from build123d import *

# Parameters (mm, degrees)
SKETCH1_W           = 177.8
SKETCH1_H           = 19.05
BOSS_EXTRUDE1_DEPTH = 3.048
CUT_EXTRUDE1_DEPTH  = 179.843598722
BOSS_EXTRUDE2_DEPTH = 3.048
FILLET1_R           = 1.5875
FILLET2_R           = 0.79375


with BuildPart() as part:
    # Sketch1 → Boss-Extrude1 (new body)
    with BuildSketch(Plane.XY):
        with Locations((-88.9, 9.525)):
            Rectangle(SKETCH1_W, SKETCH1_H)
    extrude(amount=BOSS_EXTRUDE1_DEPTH)

    # Sketch2 → Cut-Extrude1 (cut, through all)
    with BuildSketch(Plane.XY.offset(3.048)):
        with BuildLine():
            Line((-11.1125, 6.35), (-20.6375, 6.35))
            ThreePointArc((-20.6375, 6.35), (-23.8125, 9.525), (-20.6375, 12.7))
            Line((-20.6375, 12.7), (-11.1125, 12.7))
            ThreePointArc((-11.1125, 12.7), (-7.9375, 9.525), (-11.1125, 6.35))
        make_face()
        with BuildLine():
            Line((-36.5125, 6.35), (-46.0375, 6.35))
            ThreePointArc((-46.0375, 6.35), (-49.2125, 9.525), (-46.0375, 12.7))
            Line((-46.0375, 12.7), (-36.5125, 12.7))
            ThreePointArc((-36.5125, 12.7), (-33.3375, 9.525), (-36.5125, 6.35))
        make_face()
        with BuildLine():
            Line((-61.9125, 6.35), (-71.4375, 6.35))
            ThreePointArc((-71.4375, 6.35), (-74.6125, 9.525), (-71.4375, 12.7))
            Line((-71.4375, 12.7), (-61.9125, 12.7))
            ThreePointArc((-61.9125, 12.7), (-58.7375, 9.525), (-61.9125, 6.35))
        make_face()
        with BuildLine():
            Line((-87.3125, 6.35), (-96.8375, 6.35))
            ThreePointArc((-96.8375, 6.35), (-100.0125, 9.525), (-96.8375, 12.7))
            Line((-96.8375, 12.7), (-87.3125, 12.7))
            ThreePointArc((-87.3125, 12.7), (-84.1375, 9.525), (-87.3125, 6.35))
        make_face()
        with BuildLine():
            Line((-112.7125, 6.35), (-122.2375, 6.35))
            ThreePointArc((-122.2375, 6.35), (-125.4125, 9.525), (-122.2375, 12.7))
            Line((-122.2375, 12.7), (-112.7125, 12.7))
            ThreePointArc((-112.7125, 12.7), (-109.5375, 9.525), (-112.7125, 6.35))
        make_face()
        with BuildLine():
            Line((-138.1125, 6.35), (-147.6375, 6.35))
            ThreePointArc((-147.6375, 6.35), (-150.8125, 9.525), (-147.6375, 12.7))
            Line((-147.6375, 12.7), (-138.1125, 12.7))
            ThreePointArc((-138.1125, 12.7), (-134.9375, 9.525), (-138.1125, 6.35))
        make_face()
    extrude(amount=-CUT_EXTRUDE1_DEPTH, mode=Mode.SUBTRACT)

    # Sketch3 → Boss-Extrude2 (add)
    with BuildSketch(Plane(origin=(0, 0, 0), x_dir=(-1, 0, 0), z_dir=(0, 0, -1))):
        Polygon((177.8, 0), (190.5, 0), (190.5, 11.176), (177.8, 19.05), align=None)
    extrude(amount=-BOSS_EXTRUDE2_DEPTH)

    # Fillet1
    fillet1_edges = [part.edges().sort_by_distance(p)[0] for p in [
        (-190.5, 0, 1.524),
        (-190.5, 11.176, 1.524),
        (-177.8, 19.05, 1.524),
    ]]
    fillet(fillet1_edges, radius=FILLET1_R)

    # Fillet2
    fillet2_edges = [part.edges().sort_by_distance(p)[0] for p in [
        (0, 0, 1.524),
        (0, 19.05, 1.524),
    ]]
    fillet(fillet2_edges, radius=FILLET2_R)


solid = part.part
Design review of the part built by this model. Coordinates are the model's own, in mm. A direction names the side the tool comes from. Round coordinates to 2 decimals unless told otherwise and drop trailing zeros. Loops run counter-clockwise (first coordinate to the right, second up) from the corner with the lowest first, then second, coordinate; pieces in that order, holes last. Notation, with made-up numbers: M 11,41.5 L 28,41.5 A25 ccw 28,70.5 Z; hole C 37,79.5 d10. An arc over 180 degrees is marked long. Answer as a JSON object with one key per item and string values.
Item 1: We need section C-C on y = 16.25. Give the boundary of the cut face in (x, z).
Answer sheet:
{"outline": "M -182.32,0 L 0,0 L 0,3.05 L -182.32,3.05 Z"}
Item 2: We need section A-A on x = -143. Give the boundary of the cut face in (y, z), and give its area (3 significant figures).
Answer sheet:
{"outline": "M 0,0 L 6.35,0 L 6.35,3.05 L 0,3.05 Z; M 12.7,0 L 19.05,0 L 19.05,3.05 L 12.7,3.05 Z", "area": "38.7 mm^2"}
Item 3: We need section B-B on z = 0.6. State how many separate pieces and enclosed holes the cut face has, and give its area (3 significant figures).
Answer sheet:
{"separate pieces": "1", "enclosed holes": "6", "area": "3,030 mm^2"}
Item 4: The part is to be moulded in two halves that separate along Y. For faces 1 (the flat face through (-184.048, 15.176, 1.503)), 2 (the flat face through (-92, 6.35, 2)), 3 (the flat face through (-94, 14, 3.048)), say which applies: pulls with the +Y half, pulls with the -Y half, needs draft (parallel to the pull), parting line crosses it, or undercut.
Answer sheet:
{"face 1": "pulls with the +Y half", "face 2": "undercut", "face 3": "needs draft"}
Item 5: Machinability: for faces 4 (the flat face through (-90, 19.05, 2)), 5 (the flat face through (-16, 6.35, 2)), which of the approach directions +Z, -Z, +X, -X, +Y, -Y give a long, thin tool a straight path to every point of the face, cutting with its end or side? Answer none if there is none.
Answer sheet:
{"face 4": "+Z, -Z, +X, -X, +Y", "face 5": "+Z, -Z"}
Item 6: Wall thickness on L1, parallel to Y at x = -18, z = 1.35; L2, parallel to X at y = 14.25, z = 0.7: over which ranges is each line inside the solid? List them lowest first. Write a range as from..to.
Answer sheet:
{"L1": "y = 0..6.35, 12.7..19.05", "L2": "x = -185.54..0"}
